from build123d import *

# Parameters (mm, degrees)
SKETCH002_R     = 4
SKETCH002_R_2   = 1.45
SKETCH002_R_3   = 3.05
PAD002_DEPTH    = 10
SKETCH003_R     = 10.5
POCKET_DEPTH    = 7
SKETCH004_R     = 1.7
POCKET001_DEPTH = 5


with BuildPart() as part:
    # Sketch002 → Pad002 (new body)
    with BuildSketch(Plane.XY):
        with BuildLine():
            Line((-34.2875, 22), (5.7125, 22))
            Line((5.7125, 22), (12.190202, 4.516521))
            ThreePointArc((0, -13), (10.670398, -7.425807), (12.190202, 4.516521))
            Line((0, -13), (-28.575, -13))
            ThreePointArc((-40.765202, 4.516521), (-39.245398, -7.425807), (-28.575, -13))
            Line((-40.765202, 4.516521), (-34.2875, 22))
        make_face()
        Circle(SKETCH002_R, mode=Mode.SUBTRACT)
        with Locations((7.5, 0)):
            Circle(SKETCH002_R_2, mode=Mode.SUBTRACT)
        with Locations((-7.5, 0)):
            Circle(SKETCH002_R_2, mode=Mode.SUBTRACT)
        with Locations((-28.575, 0)):
            Circle(SKETCH002_R_3, mode=Mode.SUBTRACT)
    extrude(amount=PAD002_DEPTH)

    # Sketch003 → Pocket (cut)
    with BuildSketch(Plane.XY.offset(3)):
        Circle(SKETCH003_R)
    extrude(amount=POCKET_DEPTH, mode=Mode.SUBTRACT)

    # Sketch004 → Pocket001 (cut)
    with BuildSketch(Plane.XZ.offset(-22)):
        with Locations((-29.2875, 5)):
            Circle(SKETCH004_R)
        with Locations((0.7125, 5)):
            Circle(SKETCH004_R)
    extrude(amount=POCKET001_DEPTH, mode=Mode.SUBTRACT)


solid = part.part
Design review of the part built by this model. Coordinates are the model's own, in mm. A direction names the side the tool comes from. Coordinates: 2 decimals unless noted, no trailing zeros. Order: outer loops, then holes, each group sorted by start corner. A loop starts at its lowest first (then second) coordinate and runs counter-clockwise, first axis right, second up.
Item 1: Take a section at B-B, the plane y = 0. Write out the cut boundary in (x, z) (3 decimals).
Item 2: For faces 5 (the flat face through (-29, 17, 5)), 6 (the flat face through (5, 0, 3)), 7 (the flat face through (-14, 5, 0)), list the 3-axis set-ups (+Z, -Z, +X, -X, +Y, -Y) from which the entire face can be reached by the end or side of a thin tool; tool diameter is ignored.
Item 3: For pin 1 Ø10.5 at (x, y) = (0, 0) entering from +Z; pin 2 Ø3 at (x, z) = (-29.29, 5) entering from +Y; pin 3 Ø6 at (y, z) = (-6, 6) entering from +X, all flat-tipped, find the tip position at first contact; note any pin that passes through.
Item 4: For line 1 (Y direction, x = -7.5, z = 0.9); line 2 (X direction, y = -1.5, z = 8.25); line 3 (Y direction, x = 0.5, z = 8.25), list the stretches that pass through material, from the lowest coordinate up.
Item 5: Take a section at C-C, the plane x = 7.5. Write out the cut boundary in (y, z).
Item 6: Take a section at A-A, the plane z = 5. Count the separate pieces of the cut face and the enclosed holes in it, then the cut area to 3 significant figures.
Item 7: The part is to be moulded in two halves that separate along Y. For faces 1 (the cylindrical face through (10, 3.2, 6.5)), 2 (the cylindrical face through (-8.95, 0.06, 1.48)), 3 (the cylindrical face through (0.34, 19.54, 3.34)), 4 (the cylindrical face through (-39.345, -7.281, 4.93)), say which applies: pulls with the +Y half, pulls with the -Y half, needs draft (parallel to the pull), parting line crosses it, or undercut.
The answers:
1. outline: (-41.575, 0) - (-31.625, 0) - (-31.625, 10) - (-41.575, 10) - close; (-25.525, 0) - (-8.95, 0) - (-8.95, 3) - (-10.5, 3) - (-10.5, 10) - (-25.525, 10) - close; (-6.05, 0) - (-4, 0) - (-4, 3) - (-6.05, 3) - close; (4, 0) - (6.05, 0) - (6.05, 3) - (4, 3) - close; (8.95, 0) - (13, 0) - (13, 10) - (10.5, 10) - (10.5, 3) - (8.95, 3) - close
2. face 5: +Y
2. face 6: +Z
2. face 7: -Z, +X, -X, +Y, -Y
3. pin 1: stops at z = 3
3. pin 2: stops at y = 17
3. pin 3: stops at x = 12.65
4. line 1: y = -13 to -1.45, 1.45 to 22
4. line 2: x = -41.49 to -31.23, -25.92 to -10.39, 10.39 to 12.91
4. line 3: y = -12.99 to -10.49, 10.49 to 22
5. outline: (-10.62, 0) - (-1.45, 0) - (-1.45, 3) - (-7.35, 3) - (-7.35, 10) - (-10.62, 10) - close; (1.45, 0) - (17.18, 0) - (17.18, 10) - (7.35, 10) - (7.35, 3) - (1.45, 3) - close
6. separate pieces: 1
6. enclosed holes: 2
6. area: 1,280 mm2
7. face 1: undercut
7. face 2: undercut
7. face 3: needs draft
7. face 4: parting line crosses it
